```python
from build123d import *

# Parameters (mm, degrees)
SKETCH1_R           = 12
BOSS_EXTRUDE1_DEPTH = 0.85


with BuildPart() as part:
    # Sketch1 → Boss-Extrude1 (new body)
    # profile 1 of 9: a face of its own
    with BuildSketch(Plane(origin=(0, 0, 0), x_dir=(1, 0, 0), z_dir=(0, 1, 0))):
        Polygon((103.091739333, 32.005343302), (86.560327372, 32.005343302), (94.826033353, 18.229166667), align=None)
    # profile 2 of 9: a face of its own
    with BuildSketch(Plane(origin=(0, 0, 0), x_dir=(1, 0, 0), z_dir=(0, 1, 0))):
        Polygon((124.826033353, 18.229166667), (113.888533353, 0), (135.763533353, 0), align=None)
    # profile 3 of 9: a face of its own
    with BuildSketch(Plane(origin=(0, 0, 0), x_dir=(1, 0, 0), z_dir=(0, 1, 0))):
        Polygon((163.091739333, 32.005343302), (146.560327372, 32.005343302), (154.826033353, 18.229166667), align=None)
    # profile 4 of 9: a face of its own
    with BuildSketch(Plane(origin=(0, 0, 0), x_dir=(1, 0, 0), z_dir=(0, 1, 0))):
        Polygon((173.888533353, 0), (195.763533353, 0), (184.826033353, 18.229166667), align=None)
    # profile 5 of 9: a face of its own
    with BuildSketch(Plane(origin=(0, 0, 0), x_dir=(1, 0, 0), z_dir=(0, 1, 0))):
        Polygon((214.826033353, 18.229166667), (223.091739333, 32.005343302), (206.560327372, 32.005343302), align=None)
    # profile 6 of 9: a face of its own
    with BuildSketch(Plane(origin=(0, 0, 0), x_dir=(1, 0, 0), z_dir=(0, 1, 0))):
        Polygon((229.826033353, 43.229166667), (79.826033353, 43.229166667), (79.826033353, 32.005343302), (86.560327372, 32.005343302), (103.091739333, 32.005343302), (109.826033353, 32.005343302), (116.560327372, 32.005343302), (133.091739333, 32.005343302), (139.826033353, 32.005343302), (146.560327372, 32.005343302), (163.091739333, 32.005343302), (169.826033353, 32.005343302), (176.560327372, 32.005343302), (193.091739333, 32.005343302), (199.826033353, 32.005343302), (206.560327372, 32.005343302), (223.091739333, 32.005343302), (229.826033353, 32.005343302), align=None)
    # profile 7 of 9: a face of its own
    with BuildSketch(Plane(origin=(0, 0, 0), x_dir=(1, 0, 0), z_dir=(0, 1, 0))):
        Polygon((79.826033353, 0), (79.826033353, -6.770833333), (229.826033353, -6.770833333), (229.826033353, 0), (225.763533353, 0), (203.888533353, 0), (199.826033353, 0), (195.763533353, 0), (173.888533353, 0), (169.826033353, 0), (165.763533353, 0), (143.888533353, 0), (139.826033353, 0), (135.763533353, 0), (113.888533353, 0), (109.826033353, 0), (105.763533353, 0), (83.888533353, 0), align=None)
    # profile 8 of 9: a face of its own
    with BuildSketch(Plane(origin=(0, 0, 0), x_dir=(1, 0, 0), z_dir=(0, 1, 0))):
        with BuildLine():
            Line((79.826033353, 43.229166667), (35.416666667, 43.229166667))
            ThreePointArc((35.416666667, 43.229166667), (10.416666667, 18.229166667), (35.416666667, -6.770833333))
            Line((35.416666667, -6.770833333), (79.826033353, -6.770833333))
            Line((79.826033353, -6.770833333), (79.826033353, 0))
            Line((79.826033353, 0), (79.826033353, 32.005343302))
            Line((79.826033353, 32.005343302), (79.826033353, 43.229166667))
        make_face()
        with Locations(Location((49.297410929, 18.229166667, 0), (0, 0, 270))):
            Circle(SKETCH1_R, mode=Mode.SUBTRACT)
    # profile 9 of 9: a face of its own
    with BuildSketch(Plane(origin=(0, 0, 0), x_dir=(1, 0, 0), z_dir=(0, 1, 0))):
        with BuildLine():
            Line((285.416666667, 43.229166667), (229.826033353, 43.229166667))
            Line((229.826033353, 43.229166667), (229.826033353, 32.005343302))
            Line((229.826033353, 32.005343302), (229.826033353, 0))
            Line((229.826033353, 0), (229.826033353, -6.770833333))
            Line((229.826033353, -6.770833333), (285.416666667, -6.770833333))
            ThreePointArc((285.416666667, -6.770833333), (310.416666667, 18.229166667), (285.416666667, 43.229166667))
        make_face()
        with Locations(Location((264.825532318, 18.229166667, 0), (0, 0, 270))):
            Circle(SKETCH1_R, mode=Mode.SUBTRACT)
    extrude(amount=BOSS_EXTRUDE1_DEPTH)


solid = part.part
```
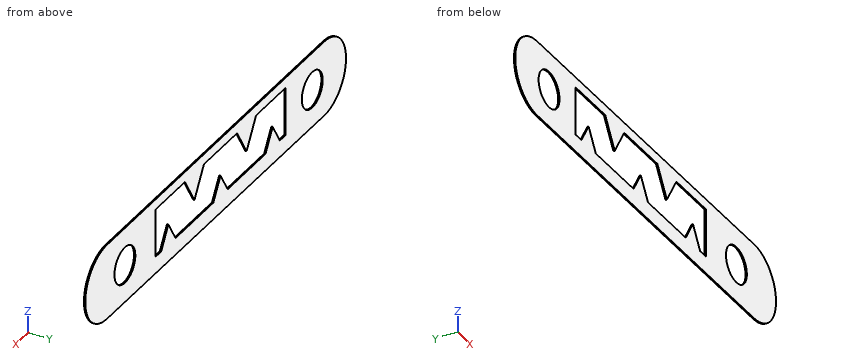
Here's how the part is built. I have some questions about the finished solid (model axes, mm). Coordinates: 2 decimals unless noted, no trailing zeros. Order: outer loops, then holes, each group sorted by start corner. A loop starts at its lowest first (then second) coordinate and runs counter-clockwise, first axis right, second up.
Item 1: If we section it at B-B, the plane y = 0.6: List the corners of the cut face in (x, z) for me, then the cut area to 3 significant figures.
Response values:
outline: (35.42, -43.23) - (285.42, -43.23) arc R25 ccw to (285.42, 6.77) - (35.42, 6.77) arc R25 ccw to start; hole circle Ø24 at (49.3, -18.23); hole (79.83, -32.01) - (86.56, -32.01) - (94.83, -18.23) - (103.09, -32.01) - (146.56, -32.01) - (154.83, -18.23) - (163.09, -32.01) - (206.56, -32.01) - (214.83, -18.23) - (223.09, -32.01) - (229.83, -32.01) - (229.83, 0) - (195.76, 0) - (184.83, -18.23) - (173.89, 0) - (135.76, 0) - (124.83, -18.23) - (113.89, 0) - (79.83, 0) - close; hole circle Ø24 at (264.83, -18.23)
area: 9,500 mm2
Item 2: I need wall thicknesses on probe 1 along X at (y, z) = (0.25, -17); probe 2 along Z at (x, y) = (229.5, 0.4); probe 3 along X at (y, z) = (0.2, -8). Which ranges of each line are inside material? Lowest first, please.
Response values:
probe 1: x = 10.45 to 37.36, 61.23 to 79.83, 124.09 to 125.56, 184.09 to 185.56, 229.83 to 252.89, 276.76 to 310.39
probe 2: z = -43.23 to -32.01, 0 to 6.77
probe 3: x = 12.61 to 43.02, 55.57 to 79.83, 118.69 to 130.96, 178.69 to 190.96, 229.83 to 258.55, 271.1 to 308.23
Item 3: If we section it at A-A, the plane z = -23: List the corners of the cut face in (x, y) for me, then the cut area to 3 significant figures.
Response values:
outline: (10.88, 0) - (38.29, 0) - (38.29, 0.85) - (10.88, 0.85) - close; (60.31, 0) - (79.83, 0) - (79.83, 0.85) - (60.31, 0.85) - close; (91.96, 0) - (97.69, 0) - (97.69, 0.85) - (91.96, 0.85) - close; (151.96, 0) - (157.69, 0) - (157.69, 0.85) - (151.96, 0.85) - close; (211.96, 0) - (217.69, 0) - (217.69, 0.85) - (211.96, 0.85) - close; (229.83, 0) - (253.81, 0) - (253.81, 0.85) - (229.83, 0.85) - close; (275.84, 0) - (309.96, 0) - (309.96, 0.85) - (275.84, 0.85) - close
area: 104 mm2
